The model under review builds one solid part; all positions refer to its coordinate system, in mm. Face numbers are marked on the shaded views. Round coordinates to 2 decimals unless told otherwise and drop trailing zeros. Loops run counter-clockwise (first coordinate to the right, second up) from the corner with the lowest first, then second, coordinate; pieces in that order, holes last. Notation, with made-up numbers: (-4, 76) -> (36, 76) arc R31 cw to (36, 105) -> close; hole circle Ø7 at (-8, 45.5). An arc over 180 degrees is marked (long way). Use CSV: the item, a comma, the result in double quotes. Start each with the question number.
```python
from build123d import *

# Parameters (mm, degrees)
SKETCH_1_W          = 150
SKETCH_1_H          = 207
EXTRUDE_1_DEPTH     = 4
CUT_EXTRUDE_1_DEPTH = 5
SKETCH_3_R          = 1.5
CUT_EXTRUDE_2_DEPTH = 5


with BuildPart() as part:
    # 草图1 → 凸台-拉伸1 (new body)
    with BuildSketch(Plane(origin=(0, 0, 0), x_dir=(1, 0, 0), z_dir=(0, 1, 0))):
        with Locations((75, 103.5)):
            Rectangle(SKETCH_1_W, SKETCH_1_H)
    extrude(amount=EXTRUDE_1_DEPTH)

    # 草图2 → 切除-拉伸1 (cut, through all)
    with BuildSketch(Plane(origin=(0, 4, 0), x_dir=(1, 0, 0), z_dir=(0, 1, 0))):
        with BuildLine():
            Line((30, 189.5), (130, 189.5))
            ThreePointArc((130, 189.5), (136, 183.5), (130, 177.5))
            Line((130, 177.5), (30, 177.5))
            ThreePointArc((30, 177.5), (24, 183.5), (30, 189.5))
        make_face()
        with BuildLine():
            Line((30, 149.5), (130, 149.5))
            ThreePointArc((130, 149.5), (136, 143.5), (130, 137.5))
            Line((130, 137.5), (30, 137.5))
            ThreePointArc((30, 137.5), (24, 143.5), (30, 149.5))
        make_face()
        with BuildLine():
            Line((30, 97.5), (130, 97.5))
            ThreePointArc((130, 97.5), (136, 103.5), (130, 109.5))
            Line((130, 109.5), (30, 109.5))
            ThreePointArc((30, 109.5), (24, 103.5), (30, 97.5))
        make_face()
        with BuildLine():
            Line((30, 57.5), (130, 57.5))
            ThreePointArc((130, 57.5), (136, 63.5), (130, 69.5))
            Line((130, 69.5), (30, 69.5))
            ThreePointArc((30, 69.5), (24, 63.5), (30, 57.5))
        make_face()
        with BuildLine():
            Line((30, 17.5), (130, 17.5))
            ThreePointArc((130, 17.5), (136, 23.5), (130, 29.5))
            Line((130, 29.5), (30, 29.5))
            ThreePointArc((30, 29.5), (24, 23.5), (30, 17.5))
        make_face()
    extrude(amount=-CUT_EXTRUDE_1_DEPTH, mode=Mode.SUBTRACT)

    # 草图3 → 切除-拉伸2 (cut, through all)
    with BuildSketch(Plane(origin=(0, 4, 0), x_dir=(1, 0, 0), z_dir=(0, 1, 0))):
        with Locations((125, 197)):
            Circle(SKETCH_3_R)
        with Locations((75, 197)):
            Circle(SKETCH_3_R)
        with Locations((25, 197)):
            Circle(SKETCH_3_R)
        with Locations((25, 10)):
            Circle(SKETCH_3_R)
        with Locations((75, 10)):
            Circle(SKETCH_3_R)
        with Locations((125, 10)):
            Circle(SKETCH_3_R)
    extrude(amount=-CUT_EXTRUDE_2_DEPTH, mode=Mode.SUBTRACT)


solid = part.part
```
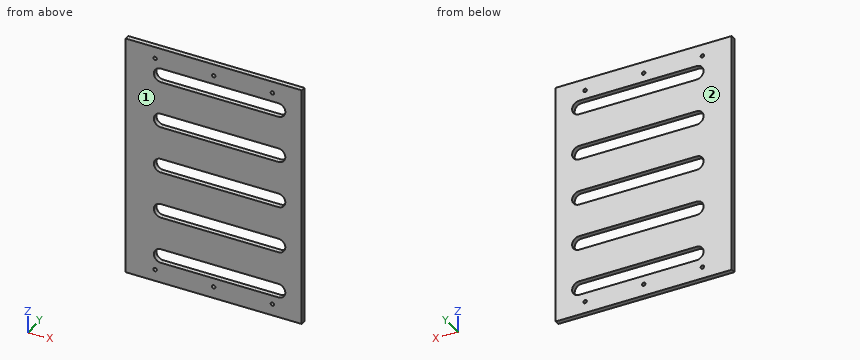
1. For line 1 along X through (y, z) = (2.45, -10); line 2 along Z through (x, y) = (70, 1.65); line 3 along X through (y, z) = (2.3, -178), list the stretches that pass through material, from the lowest coordinate up. Write a range as from..to.
2. Take a section at A-A, the plane z = -23.5. Give the boundary of the cut face in (x, y), then the cut area to 3 significant figures.
3. The part is to be moulded in two halves that separate along Y. For the marked faces 1 and 2, say which applies: pulls with the +Y half, pulls with the -Y half, needs draft (parallel to the pull), parting line crosses it, or undercut.
4. Take a section at C-C, the plane x = 58. Give the boundary of the cut face in (y, z).
5. Take a section at B-B, the plane y = 2.75. Count the separate pieces of the cut face and the enclosed holes in it, then the cut area to 3 significant figures.
Results:
1,line 1,"0..23.5, 26.5..73.5, 76.5..123.5, 126.5..150"
1,line 2,"-207..-189.5, -177.5..-149.5, -137.5..-109.5, -97.5..-69.5, -57.5..-29.5, -17.5..0"
1,line 3,"0..27.6, 132.4..150"
2,outline,"(0, 0) -> (24, 0) -> (24, 4) -> (0, 4) -> close; (136, 0) -> (150, 0) -> (150, 4) -> (136, 4) -> close"
2,area,"152 mm²"
3,face 1,"pulls with the -Y half"
3,face 2,"pulls with the +Y half"
4,outline,"(0, -207) -> (4, -207) -> (4, -189.5) -> (0, -189.5) -> close; (0, -177.5) -> (4, -177.5) -> (4, -149.5) -> (0, -149.5) -> close; (0, -137.5) -> (4, -137.5) -> (4, -109.5) -> (0, -109.5) -> close; (0, -97.5) -> (4, -97.5) -> (4, -69.5) -> (0, -69.5) -> close; (0, -57.5) -> (4, -57.5) -> (4, -29.5) -> (0, -29.5) -> close; (0, -17.5) -> (4, -17.5) -> (4, 0) -> (0, 0) -> close"
5,separate pieces,"1"
5,enclosed holes,"11"
5,area,"24,400 mm²"
